Drawing for the job (mm, zero at the part's lowest x, y, z). A direction names the side the tool comes from. Round coordinates to 2 decimals unless told otherwise and drop trailing zeros. Order: outer loops, then holes, each group sorted by start corner. A loop starts at its lowest first (then second) coordinate and runs counter-clockwise, first axis right, second up. Notation, with made-up numbers: M 4.5,4 L 30.5,4 A19 cw 30.5,31 Z; hole C 2,78.5 d4. An arc over 180 degrees is marked long. One line per item, written item: value. Start each with the question number.
Item 1: Two-plate mould, pull along Z, no slides. Class the marked faces 4, 5 and 6: +Z half, -Z half, draft (parallel to the pull), parting line (faces both ways), or undercut.
Item 2: Band-saw the part on D-D, the plane x = 6.5. Write the cut outline in (y, z).
Item 3: Probe L1, parallel to Y at x = 10, z = 2.95; L2, parallel to Z at x = 5, y = 10; L3, parallel to Y at x = 18.75, z = 9. List the from-to ranges inside material, lowest first.
Item 4: Tool access for the marked faces 1, 2 and 3: list every direction of +Z, -Z, +X, -X, +Y, -Y with a clear straight run to the whole face (end or side of a thin tool).
Item 5: Band-saw the part on B-B, the plane x = 10. Write the cut outline in (y, z), then the cut area to 3 significant figures.
Item 6: Pin check, flat tip, straight feed: pin 1 (4 mm diameter, centred on x = 6, y = 42.5, fed in from +Z). Stop position of the tip, or through.
Item 7: Band-saw the part on A-A, the plane y = 6.5. Write the cut outline in (x, z), then the cut area to 3 significant figures.
Item 8: Band-saw the part on C-C, the plane z = 20. Write the cut outline in (x, y), then the cut area to 3 significant figures.
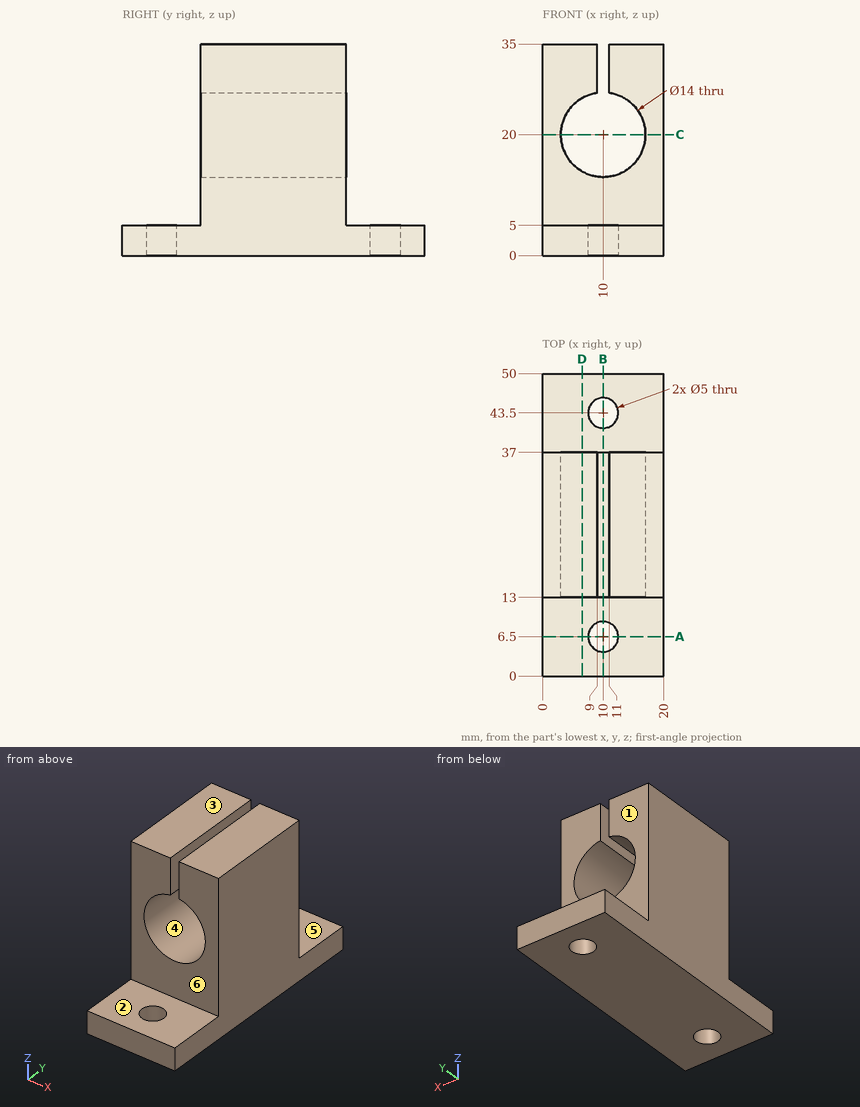
Output:
1. face 4: undercut
1. face 5: +Z half
1. face 6: draft
2. outline: M 0,0 L 50,0 L 50,5 L 37,5 L 37,13.94 L 13,13.94 L 13,5 L 0,5 Z; M 13,26.06 L 37,26.06 L 37,35 L 13,35 Z
3. L1: y = 0 to 4, 9 to 41, 46 to 50
3. L2: z = 0 to 5
3. L3: y = 13 to 37
4. face 1: +Z, +X, -X, +Y
4. face 2: +Z, +X, -X, -Y
4. face 3: +Z, +X, -X, +Y, -Y
5. outline: M 0,0 L 4,0 L 4,5 L 0,5 Z; M 9,0 L 41,0 L 41,5 L 37,5 L 37,13 L 13,13 L 13,5 L 9,5 Z; M 46,0 L 50,0 L 50,5 L 46,5 Z
5. area: 392 mm²
6. pin 1: stops at z = 5
7. outline: M 0,0 L 7.5,0 L 7.5,5 L 0,5 Z; M 12.5,0 L 20,0 L 20,5 L 12.5,5 Z
7. area: 75.0 mm²
8. outline: M 0,13 L 3,13 L 3,37 L 0,37 Z; M 17,13 L 20,13 L 20,37 L 17,37 Z
8. area: 144 mm²
